Work out the finished part from the listing and answer in its coordinate system (mm). Face numbers are marked on the shaded views. A direction names the side the tool comes from. Coordinates: 2 decimals unless noted, no trailing zeros. Loops run counter-clockwise (first coordinate to the right, second up) from the corner with the lowest first, then second, coordinate; pieces in that order, holes last. Notation, with made-up numbers: (6.25, -20) - (34.25, -20) arc R15 cw to (34.25, -15) - close; hole circle Ø10 at (88.5, 8). An arc over 180 degrees is marked (long way). Write each question's results on one line, items separated by ' | '. Start each with the question number.
Item 1: Each of these flat-tipped pins is pushed along its axis until it touches: pin 1 Ø1 at (y, z) = (-59, 13.5) entering from +X; pin 2 Ø10.5 at (x, y) = (36.5, 31) entering from +Z; pin 3 Ø1.5 at (y, z) = (56, 13.5) entering from -X. Where does it stop, or does it pass through?
Item 2: Consider probe 1 along X at (y, z) = (30, 26); probe 2 along X at (y, z) = (30, 28); probe 3 along Y at (x, z) = (-30, 26). Determine where each line is inside the solid, lowest interval first. Write a range as [from, to].
Item 3: Section B-B, the plane z = 25 is taken. Write down the section's boundary in (x, y).
Item 4: A tool of negligible diameter and unlimited length cuts with its end or side. For the marked faces 4, 5 and 6, from which of +Z, -Z, +X, -X, +Y, -Y can it reach the whole face along a straight path? Write none if from no direction.
Item 5: For a pull along X with two mould halves and no side action, classify the marked faces 1, 2 and 3 as +X half, -X half, draft (parallel to the pull), parting line (faces both ways), or undercut.
Item 6: Section A-A, the plane z = 7.5 is taken. Write down the section's boundary in (x, y).
Autodesk Fusion 360 part; units mm, degrees
sketch "Sketch1" plane through (0, 0, 0) normal (0, 0, 1) x (1, 0, 0)
  line L0 (-75, 75) -> (75, 75)
  line L1 (75, 75) -> (75, -75)
  line L2 (75, -75) -> (-75, -75)
  line L3 (-75, -75) -> (-75, 75)
  line L4 (-75, 75) -> (75, -75) construction
  line L5 (75, 75) -> (-75, -75) construction
  dimension "d1" = 150
  dimension "d2" = 150
extrude "Extrude1" add sketch "Sketch1" along normal blind 10
sketch "Sketch2" plane through (0, 0, 10) normal (0, 0, 1) x (-1, 0, 0)
  line L0 (75, 75) -> (-75, 75)
  line L1 (-75, 75) -> (-75, -75)
  line L2 (-75, -75) -> (75, -75)
  line L3 (75, -75) -> (75, 75)
  circle A0 centre (0, 0) radius 75
extrude "Extrude2" add sketch "Sketch2" along normal blind 20 contours A0
sketch "Sketch3" plane through (0, 0, 30) normal (0, 0, 1) x (-1, 0, 0)
  circle A0 centre (0, 0) radius 75
  circle A1 centre (-30, -30) radius 17.5
  line L0 (0, -2.5) -> (0, -20)
  circle A2 centre (30, -30) radius 17.5
  arc A3 (36.9231, 22.8846) -> (-36.9231, 22.8846) centre (0, 7.5) ccw
  arc A4 (23.0769, 17.1154) -> (36.9231, 22.8846) centre (30, 20) ccw
  arc A5 (23.0769, 17.1154) -> (-23.0769, 17.1154) centre (0, 7.5) ccw
  arc A6 (-36.9231, 22.8846) -> (-23.0769, 17.1154) centre (-30, 20) ccw
  arc A7 (30, 20) -> (-30, 20) centre (0, 7.5) ccw construction
  dimension "d7" = 35
  dimension "d8" = 15
extrude "Extrude3" cut sketch "Sketch3" against normal blind 10 contours A1 | A2 | A3 A4 A5 A6
chamfer "Chamfer1" distance 20 angle 45 4 edges at (75, 75, 5) (75, -75, 5) (-75, -75, 5) (-75, 75, 5)
fillet "Fillet1" radius 10 1 edges at (69.9246, 27.1212, 30)
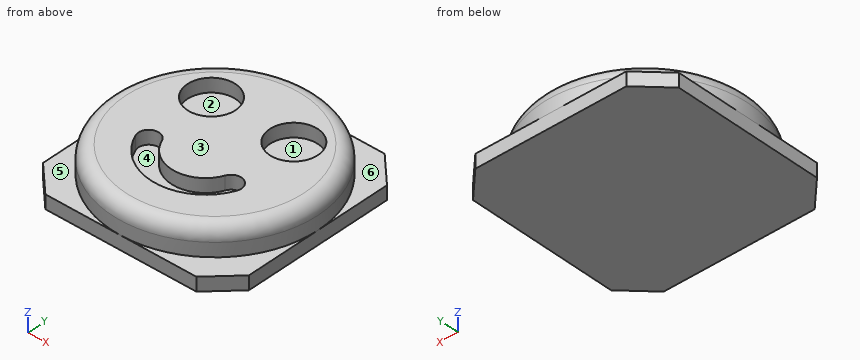
Answer key:
1) pin 1: stops at x = 46.93 | pin 2: stops at z = 20 | pin 3: stops at x = -50.72
2) probe 1: x = [-66.55, -47.5], [-12.5, 12.5], [47.5, 66.55] | probe 2: x = [-64.35, -47.5], [-12.5, 12.5], [47.5, 64.35] | probe 3: y = [-66.55, -33.96], [-12.5, 12.5], [47.5, 66.55]
3) outline: circle Ø147.32 at (0, 0); hole circle Ø35 at (-30, 30); hole (-36.92, -22.88) arc R40 ccw to (36.92, -22.88) arc R7.5 ccw to (23.08, -17.12) arc R25 cw to (-23.08, -17.12) arc R7.5 ccw to start; hole circle Ø35 at (30, 30)
4) face 4: +Z | face 5: +Z, -X, -Y | face 6: +Z, +X, +Y
5) face 1: undercut | face 2: undercut | face 3: draft
6) outline: (-75, -55) - (-55, -75) - (55, -75) - (75, -55) - (75, 55) - (55, 75) - (-55, 75) - (-75, 55) - close
